Geometry: final body of the model. Coordinates: model frame, mm. Face numbers are marked on the shaded views. A direction names the side the tool comes from. Round coordinates to 2 decimals unless told otherwise and drop trailing zeros. Loops run counter-clockwise (first coordinate to the right, second up) from the corner with the lowest first, then second, coordinate; pieces in that order, holes last. Notation, with made-up numbers: (82.5, 88.5) -> (141.5, 88.5) arc R9 cw to (141.5, 99.5) -> close; hole circle Ø7 at (78.5, -19.5). An arc over 180 degrees is marked (long way). Answer in a Markdown table with one row per item.
```python
from build123d import *

# Parameters (mm, degrees)
SKETCH1_W           = 35
SKETCH1_H           = 49
BOSS_EXTRUDE1_DEPTH = 17
SKETCH2_R           = 2
CUT_EXTRUDE1_DEPTH  = 37
SKETCH3_W           = 17
SKETCH3_H           = 35.5
BOSS_EXTRUDE2_DEPTH = 9
SKETCH4_W           = 17
SKETCH4_H           = 35.5
BOSS_EXTRUDE3_DEPTH = 9
CUT_EXTRUDE2_DEPTH  = 59
SKETCH6_R           = 6.25
CUT_EXTRUDE3_DEPTH  = 5
CUT_EXTRUDE4_START  = -5
SKETCH7_R           = 6.25
CUT_EXTRUDE4_DEPTH  = 5
SKETCH8_R           = 6.25
CUT_EXTRUDE5_DEPTH  = 5
CUT_EXTRUDE6_START  = -5
SKETCH9_R           = 6.25
CUT_EXTRUDE6_DEPTH  = 5
SKETCH10_R          = 4
BOSS_EXTRUDE4_DEPTH = 0.5
CUT_EXTRUDE7_DEPTH  = 5
CUT_EXTRUDE8_START  = -5
CUT_EXTRUDE8_DEPTH  = 5
CUT_EXTRUDE9_DEPTH  = 5
CUT_EXTRUDE10_START = -5
CUT_EXTRUDE10_DEPTH = 5
SKETCH15_R          = 6
BOSS_EXTRUDE5_DEPTH = 15
SKETCH19_R          = 2
CUT_EXTRUDE11_DEPTH = 24


with BuildPart() as part:
    # Sketch1 → Boss-Extrude1 (new body)
    with BuildSketch(Plane(origin=(0, 0, 0), x_dir=(0, 0, -1), z_dir=(1, 0, 0))):
        with Locations((17.5, 24.5)):
            Rectangle(SKETCH1_W, SKETCH1_H)
    extrude(amount=BOSS_EXTRUDE1_DEPTH)

    # Sketch2 → Cut-Extrude1 (cut)
    with BuildSketch(Plane(origin=(17, 0, 0), x_dir=(0, 0, -1), z_dir=(1, 0, 0))):
        with Locations((9, 43)):
            Circle(SKETCH2_R)
        with Locations((26, 43)):
            Circle(SKETCH2_R)
    extrude(amount=-CUT_EXTRUDE1_DEPTH, mode=Mode.SUBTRACT)

    # Sketch3 → Boss-Extrude2 (add)
    with BuildSketch(Plane(origin=(17, 0, 0), x_dir=(0, 0, -1), z_dir=(1, 0, 0))):
        with Locations((17.5, 17.75)):
            Rectangle(SKETCH3_W, SKETCH3_H)
    extrude(amount=BOSS_EXTRUDE2_DEPTH)

    # Sketch4 → Boss-Extrude3 (add)
    with BuildSketch(Plane.ZY):
        with Locations((-17.5, 17.75)):
            Rectangle(SKETCH4_W, SKETCH4_H)
    extrude(amount=BOSS_EXTRUDE3_DEPTH)

    # Sketch5 → Cut-Extrude2 (cut)
    with BuildSketch(Plane.XY):
        with BuildLine():
            Line((17, 35.5), (13.822875656, 35.5))
            ThreePointArc((13.822875656, 35.5), (10.5, 37), (13.822875656, 38.5))
            Line((13.822875656, 38.5), (17, 38.5))
            Line((17, 38.5), (17, 35.5))
        make_face()
    extrude(amount=-CUT_EXTRUDE2_DEPTH, mode=Mode.SUBTRACT)

    # Sketch6 → Cut-Extrude3 (cut)
    with BuildSketch(Plane(origin=(26, 0, 0), x_dir=(0, 0, -1), z_dir=(1, 0, 0))):
        with Locations((17.5, 28.25)):
            Circle(SKETCH6_R)
    extrude(amount=-CUT_EXTRUDE3_DEPTH, mode=Mode.SUBTRACT)

    # Sketch7 → Cut-Extrude4 (cut)
    with BuildSketch(Plane.ZY.offset(9).offset(CUT_EXTRUDE4_START)):
        with Locations(Location((-17.5, 28.25, 0), (0, 0, 180))):
            Circle(SKETCH7_R)
    extrude(amount=CUT_EXTRUDE4_DEPTH, mode=Mode.SUBTRACT)

    # Sketch8 → Cut-Extrude5 (cut)
    with BuildSketch(Plane(origin=(0, 0, -35), x_dir=(-1, 0, 0), z_dir=(0, 0, -1))):
        with Locations(Location((-8.5, 28.25, 0), (0, 0, 90))):
            Circle(SKETCH8_R)
    extrude(amount=-CUT_EXTRUDE5_DEPTH, mode=Mode.SUBTRACT)

    # Sketch9 → Cut-Extrude6 (cut)
    with BuildSketch(Plane.XY.offset(CUT_EXTRUDE6_START)):
        with Locations(Location((8.5, 28.25, 0), (0, 0, 90))):
            Circle(SKETCH9_R)
    extrude(amount=CUT_EXTRUDE6_DEPTH, mode=Mode.SUBTRACT)

    # Sketch10 → Boss-Extrude4 (add)
    with BuildSketch(Plane(origin=(17, 0, 0), x_dir=(0, 0, -1), z_dir=(1, 0, 0))):
        with Locations(Location((17.5, 43, 0), (0, 0, 180))):
            Circle(SKETCH10_R)
        Polygon((18.636585466, 44.653193152), (16.636585466, 44.810908463), (15.5, 43.157715311), (16.363414534, 41.346806848), (18.363414534, 41.189091537), (19.5, 42.842284689), align=None, mode=Mode.SUBTRACT)
    extrude(amount=BOSS_EXTRUDE4_DEPTH)

    # Sketch11 → Cut-Extrude7 (cut)
    with BuildSketch(Plane(origin=(26, 0, 0), x_dir=(0, 0, -1), z_dir=(1, 0, 0))):
        with BuildLine():
            Line((13.5, 0), (21.5, 0))
            Line((21.5, 0), (21.5, 16))
            ThreePointArc((21.5, 16), (17.5, 20), (13.5, 16))
            Line((13.5, 16), (13.5, 0))
        make_face()
    extrude(amount=-CUT_EXTRUDE7_DEPTH, mode=Mode.SUBTRACT)

    # Sketch12 → Cut-Extrude8 (cut)
    with BuildSketch(Plane.ZY.offset(9).offset(CUT_EXTRUDE8_START)):
        with BuildLine():
            Line((-21.5, 0), (-13.5, 0))
            Line((-13.5, 0), (-13.5, 16))
            ThreePointArc((-13.5, 16), (-17.5, 20), (-21.5, 16))
            Line((-21.5, 16), (-21.5, 0))
        make_face()
    extrude(amount=CUT_EXTRUDE8_DEPTH, mode=Mode.SUBTRACT)

    # Sketch13 → Cut-Extrude9 (cut)
    with BuildSketch(Plane(origin=(0, 0, -35), x_dir=(-1, 0, 0), z_dir=(0, 0, -1))):
        with BuildLine():
            Line((-12.5, 0), (-4.5, 0))
            Line((-4.5, 0), (-4.5, 16))
            ThreePointArc((-4.5, 16), (-8.5, 20), (-12.5, 16))
            Line((-12.5, 16), (-12.5, 0))
        make_face()
    extrude(amount=-CUT_EXTRUDE9_DEPTH, mode=Mode.SUBTRACT)

    # Sketch14 → Cut-Extrude10 (cut)
    with BuildSketch(Plane.XY.offset(CUT_EXTRUDE10_START)):
        with BuildLine():
            Line((4.5, 0), (12.5, 0))
            Line((12.5, 0), (12.5, 16))
            ThreePointArc((12.5, 16), (8.5, 20), (4.5, 16))
            Line((4.5, 16), (4.5, 0))
        make_face()
    extrude(amount=CUT_EXTRUDE10_DEPTH, mode=Mode.SUBTRACT)

    # Sketch15 → Boss-Extrude5 (add)
    with BuildSketch(Plane(origin=(0, 49, 0), x_dir=(1, 0, 0), z_dir=(0, 1, 0))):
        with Locations(Location((8.5, 17.5, 0), (0, 0, 270))):
            Circle(SKETCH15_R)
    extrude(amount=BOSS_EXTRUDE5_DEPTH)

    # Sketch19 → Cut-Extrude11 (cut)
    with BuildSketch(Plane(origin=(0, 64, 0), x_dir=(1, 0, 0), z_dir=(0, 1, 0))):
        with Locations(Location((8.5, 17.5, 0), (0, 0, 270))):
            Circle(SKETCH19_R)
    extrude(amount=-CUT_EXTRUDE11_DEPTH, mode=Mode.SUBTRACT)


solid = part.part
```
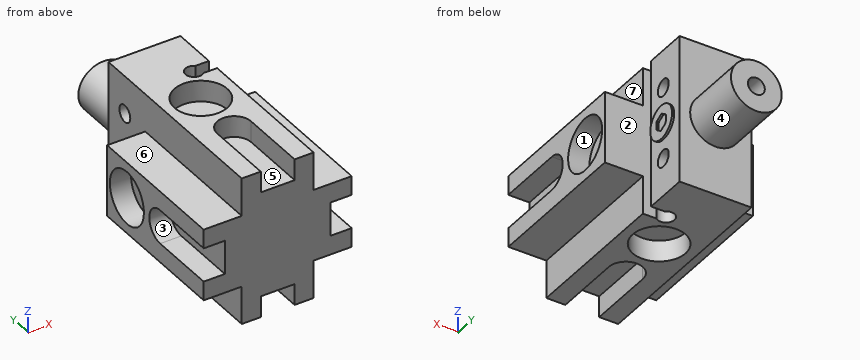
Item 1: Cut plane A-A (x = 15.5). Output: boundary loops of the cut face in (y, z), then the cut area to 3 significant figures.
Answer:
| item | result |
|---|---|
| outline | (0, -35) -> (35.5, -35) -> (35.5, 0) -> (0, 0) -> close; (38.5, -35) -> (49, -35) -> (49, 0) -> (38.5, 0) -> close; hole circle Ø4 at (43, -26); hole circle Ø4 at (43, -9) |
| area | 1,580 mm² |
Item 2: Line query: probe 1 along Y at (x, z) = (6, -26); probe 2 along X at (y, z) = (47.75, -17.5); probe 3 along X at (y, z) = (28.25, -1.2). Output: solid intervals per line, ascending. Write a range as [from, to].
Answer:
| item | result |
|---|---|
| probe 1 | y = [0, 41], [45, 49] |
| probe 2 | x = [0, 6.5], [10.5, 17] |
| probe 3 | x = [0, 2.25], [14.75, 17] |
Item 3: Draft query along X for the marked faces 5, 6 and 7. Return one class per face: pulls with the +X half, pulls with the -X half, needs draft (parallel to the pull), parting line crosses it, or undercut.
Answer:
| item | result |
|---|---|
| face 5 | undercut |
| face 6 | needs draft |
| face 7 | pulls with the +X half |
Item 4: Reachability of the marked faces 1, 2, 3 and 4 from +Z, -Z, +X, -X, +Y, -Y: full face, straight path, thin tool, end or side. Return the list, or none.
Answer:
| item | result |
|---|---|
| face 1 | +X |
| face 2 | +Z, -Z, +X |
| face 3 | -X, -Y |
| face 4 | +Y |
Item 5: Pin query (flat end, axial travel): pin 1 Ø2.5 at (y, z) = (10, -1.5) entering from +X; pin 2 Ø3 at (y, z) = (43.5, -18.5) entering from +X; pin 3 Ø1 at (x, z) = (14.5, -9) entering from +Y; pin 4 Ø4 at (y, z) = (20.5, -8.5) entering from +X. Return the tip coordinate at first contact, or that it passes through.
Answer:
| item | result |
|---|---|
| pin 1 | stops at x = 17 |
| pin 2 | stops at x = 17.5 |
| pin 3 | stops at y = 49 |
| pin 4 | stops at x = 26 |
Item 6: Cut plane B-B (x = 8.5). Output: boundary loops of the cut face in (y, z), then the cut area to 3 significant figures.
Answer:
| item | result |
|---|---|
| outline | (0, -30) -> (20, -30) -> (20, -35) -> (22, -35) -> (22, -30) -> (34.5, -30) -> (34.5, -35) -> (49, -35) -> (49, -23.5) -> (64, -23.5) -> (64, -19.5) -> (40, -19.5) -> (40, -15.5) -> (64, -15.5) -> (64, -11.5) -> (49, -11.5) -> (49, 0) -> (34.5, 0) -> (34.5, -5) -> (22, -5) -> (22, 0) -> (20, 0) -> (20, -5) -> (0, -5) -> close; hole circle Ø4 at (43, -26); hole circle Ø4 at (43, -9) |
| area | 1,450 mm² |
Item 7: Cut plane C-C (y = 12). Output: boundary loops of the cut face in (x, z), then the cut area to 3 significant figures.
Answer:
| item | result |
|---|---|
| outline | (-9, -26) -> (0, -26) -> (0, -35) -> (4.5, -35) -> (4.5, -30) -> (12.5, -30) -> (12.5, -35) -> (17, -35) -> (17, -26) -> (26, -26) -> (26, -21.5) -> (21, -21.5) -> (21, -13.5) -> (26, -13.5) -> (26, -9) -> (17, -9) -> (17, 0) -> (12.5, 0) -> (12.5, -5) -> (4.5, -5) -> (4.5, 0) -> (0, 0) -> (0, -9) -> (-9, -9) -> (-9, -13.5) -> (-4, -13.5) -> (-4, -21.5) -> (-9, -21.5) -> close |
| area | 741 mm² |
Item 8: Cut plane D-D (x = 24). Output: boundary loops of the cut face in (y, z).
Answer:
| item | result |
|---|---|
| outline | (0, -26) -> (35.5, -26) -> (35.5, -9) -> (0, -9) -> (0, -13.5) -> (16, -13.5) arc R4 cw to (16, -21.5) -> (0, -21.5) -> close; hole circle Ø12.5 at (28.25, -17.5) |
